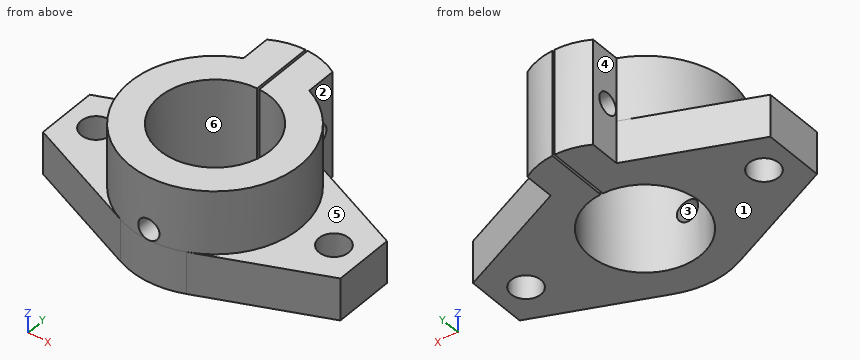
```python
from build123d import *

# Parameters (mm, degrees)
SKETCH_1_R          = 3.5
SKETCH_1_R_2        = 13
EXTRUDE_2_DEPTH     = 10
SKETCH_2_R          = 13
EXTRUDE_3_DEPTH     = 15
SKETCH_3_W          = 0.517195108
SKETCH_3_H          = 18.726193104
CUT_EXTRUDE_1_DEPTH = 26
SKETCH_4_R          = 2.5
CUT_EXTRUDE_2_DEPTH = 43.740275714
SKETCH_5_R          = 2.5
CUT_EXTRUDE_3_DEPTH = 21


with BuildPart() as part:
    # 草图1 → 凸台-拉伸2 (new body)
    with BuildSketch(Plane.XY):
        with BuildLine():
            Line((-35, -7), (-7.740275714, -18.44147857))
            ThreePointArc((-7.740275714, -18.44147857), (0, -20), (7.740275714, -18.44147857))
            Line((7.740275714, -18.44147857), (35, -7))
            Line((35, -7), (35, 7))
            Line((35, 7), (7.740275714, 18.44147857))
            Line((7.740275714, 18.44147857), (7.740275714, 25.44147857))
            ThreePointArc((7.740275714, 25.44147857), (0, 27.494244152), (-7.740275714, 25.44147857))
            Line((-7.740275714, 25.44147857), (-7.740275714, 18.44147857))
            Line((-7.740275714, 18.44147857), (-35, 7))
            Line((-35, 7), (-35, -7))
        make_face()
        with Locations((-28, 0)):
            Circle(SKETCH_1_R, mode=Mode.SUBTRACT)
        Circle(SKETCH_1_R_2, mode=Mode.SUBTRACT)
        with Locations((28, 0)):
            Circle(SKETCH_1_R, mode=Mode.SUBTRACT)
    extrude(amount=EXTRUDE_2_DEPTH)

    # 草图2 → 凸台-拉伸3 (add)
    with BuildSketch(Plane.XY.offset(10)):
        with BuildLine():
            Line((-7.740275714, 18.44147857), (-7.740275714, 25.44147857))
            ThreePointArc((-7.740275714, 25.44147857), (0, 27.494244152), (7.740275714, 25.44147857))
            Line((7.740275714, 25.44147857), (7.740275714, 18.44147857))
            ThreePointArc((7.740275714, 18.44147857), (0, -20), (-7.740275714, 18.44147857))
        make_face()
        Circle(SKETCH_2_R, mode=Mode.SUBTRACT)
    extrude(amount=EXTRUDE_3_DEPTH)

    # 草图3 → 切除-拉伸1 (cut, through all)
    with BuildSketch(Plane.XY.offset(25)):
        with Locations((0, 21.741202931)):
            Rectangle(SKETCH_3_W, SKETCH_3_H)
    extrude(amount=-CUT_EXTRUDE_1_DEPTH, mode=Mode.SUBTRACT)

    # 草图4 → 切除-拉伸2 (cut, through all)
    with BuildSketch(Plane(origin=(7.740275714, 0, 0), x_dir=(0, 0, -1), z_dir=(1, 0, 0))):
        with Locations((-12.5, 21.086423576)):
            Circle(SKETCH_4_R)
    extrude(amount=-CUT_EXTRUDE_2_DEPTH, mode=Mode.SUBTRACT)

    # 草图5 → 切除-拉伸3 (cut, through all)
    with BuildSketch(Plane(origin=(0, 0, 0), x_dir=(1, 0, 0), z_dir=(0, 1, 0))):
        with Locations((0, -12.5)):
            Circle(SKETCH_5_R)
    extrude(amount=-CUT_EXTRUDE_3_DEPTH, mode=Mode.SUBTRACT)


solid = part.part
```
Verification items for the finished model (mm, model axes). Face numbers are marked on the shaded views. A direction names the side the tool comes from. Round coordinates to 2 decimals unless told otherwise and drop trailing zeros. Order: outer loops, then holes, each group sorted by start corner. A loop starts at its lowest first (then second) coordinate and runs counter-clockwise, first axis right, second up. Notation, with made-up numbers: (74, -11) - (93, -11) arc R15 cw to (93, 13) - close; hole circle Ø11 at (3.5, 20). An arc over 180 degrees is marked (long way). Use CSV: the item, a comma, the result in double quotes. Start each with the question number.
1) Section check B-B, the plane z = 2. Record the cut outline in (x, y), plus the area to 3 significant figures.
2) Section check D-D, the plane z = 12.5. Record the cut outline in (x, y), plus the area to 3 significant figures.
3) Go/stop test with flat-tipped pins: P1, Ø5, axis at x = -5.5, z = 16.5, coming from the -Y side; P2, Ø6.5, axis at x = 28, y = 0, coming from the -Z side; P3, Ø8, axis at y = 21.09, z = 12.5, coming from the -X side; P4, Ø3.5, axis at y = 22, z = 7, coming from the -X side. Record where each tip stops, or that it passes through.
4) Access from +Z, -Z, +X, -X, +Y, -Y to the whole of each face (thin tool, end or side, straight path). Record for the marked faces 1, 2 and 3.
5) Thickness scan on L1, parallel to X at y = 0, z = 17; L2, parallel to X at y = 21, z = 1; L3, parallel to Y at x = -3.5, z = 12.5. Record the ranges inside material, lowest first.
6) Mould release check, pull along X, two halves, no side actions. Record for the marked faces 4, 5 and 6: +X half, -X half, draft (parallel to the pull), parting line (faces both ways), or undercut.
7) Section check C-C, the plane x = 27. Record the cut outline in (y, z), plus the area to 3 significant figures.
8) Section check A-A, the plane y = 0. Record the cut outline in (x, z).
Answers:
1,outline,"(-35, -7) - (-7.74, -18.44) arc R20 ccw to (7.74, -18.44) - (35, -7) - (35, 7) - (7.74, 18.44) - (7.74, 25.44) arc R15.62 ccw to (0.26, 27.49) - (0.26, 13) arc R13 cw (long way) to (-0.26, 13) - (-0.26, 27.49) arc R15.62 ccw to (-7.74, 25.44) - (-7.74, 18.44) - (-35, 7) - close; hole circle Ø7 at (-28, 0); hole circle Ø7 at (28, 0)"
1,area,"1,490 mm²"
2,outline,"(-7.74, 18.44) arc R20 ccw to (-2.5, -19.84) - (-2.5, -12.76) arc R13 cw to (-0.26, 13) - (-0.26, 18.59) - (-7.74, 18.59) - close; (-7.74, 23.59) - (-0.26, 23.59) - (-0.26, 27.49) arc R15.62 ccw to (-7.74, 25.44) - close; (0.26, 13) arc R13 cw to (2.5, -12.76) - (2.5, -19.84) arc R20 ccw to (7.74, 18.44) - (7.74, 18.59) - (0.26, 18.59) - close; (0.26, 23.59) - (7.74, 23.59) - (7.74, 25.44) arc R15.62 ccw to (0.26, 27.49) - close"
2,area,"722 mm²"
3,P1,"stops at y = -19.77"
3,P2,"passes through"
3,P3,"stops at x = -10.39"
3,P4,"stops at x = -7.74"
4,face 1,"-Z, +X, -X, +Y, -Y"
4,face 2,"+Z, -Z, +X, +Y"
4,face 3,"-Y"
5,L1,"x = -20 to -13, 13 to 20"
5,L2,"x = -7.74 to -0.26, 0.26 to 7.74"
5,L3,"y = -19.69 to -12.52, 12.52 to 18.59, 23.59 to 27.1"
6,face 4,"-X half"
6,face 5,"draft"
6,face 6,"undercut"
7,outline,"(-10.36, 0) - (-3.35, 0) - (-3.35, 10) - (-10.36, 10) - close; (3.35, 0) - (10.36, 0) - (10.36, 10) - (3.35, 10) - close"
7,area,"140 mm²"
8,outline,"(-35, 0) - (-31.5, 0) - (-31.5, 10) - (-35, 10) - close; (-24.5, 0) - (-13, 0) - (-13, 25) - (-20, 25) - (-20, 10) - (-24.5, 10) - close; (13, 0) - (24.5, 0) - (24.5, 10) - (20, 10) - (20, 25) - (13, 25) - close; (31.5, 0) - (35, 0) - (35, 10) - (31.5, 10) - close"
